```python
from build123d import *

# Parameters (mm, degrees)
F0_R     = 22.225
F1_DEPTH = 12.7
F0_R_2   = 9.525
F0_R_3   = 14.2875
F2_DEPTH = 22.225


with BuildPart() as f1:
    # F0 (on Right) → F1 (new body, symmetric)
    with BuildSketch(Plane.YZ):
        with BuildLine():
            ThreePointArc((0.7709428469, 53.3727500739), (1.3823409605, 50.5277313214), (1.5875, 47.625))
            ThreePointArc((1.5875, 47.625), (-21.5859879765, 27.1439069815), (-39.0642428209, 52.6585365854))
            ThreePointArc((-39.0642428209, 52.6585365854), (-54.8414617427, 28.4450035745), (-82.1718427428, 19.05))
            Line((-82.1718427428, 19.05), (-63.2968, 19.05))
            ThreePointArc((-63.2968, 19.05), (-44.2468, 0), (-63.2968, -19.05))
            Line((-63.2968, -19.05), (-88.6968, -19.05))
            ThreePointArc((-88.6968, -19.05), (-90.408513446, -18.9729422357), (-92.1063790378, -18.7423923442))
            Line((-92.1063790378, -18.7423923442), (-6.2508949026, -34.3610526311))
            ThreePointArc((-6.2508949026, -34.3610526311), (12.8175803312, -32.4879248253), (28.0282905638, -20.8367596586))
            ThreePointArc((28.0282905638, -20.8367596586), (37.6405240223, -14.7442138944), (48.8602257395, -16.650109833))
            ThreePointArc((48.8602257395, -16.650109833), (68.3067503871, -16.8143453506), (78.0777321497, 0))
            ThreePointArc((78.0777321497, 0), (73.3690687488, 26.7041571404), (59.8110128446, 50.1873988183))
            ThreePointArc((59.8110128446, 50.1873988183), (44.0883532808, 57.07968597), (29.0718597616, 48.7603970384))
            ThreePointArc((29.0718597616, 48.7603970384), (13.4642776808, 42.1258150573), (0.7709428469, 53.3727500739))
        make_face()
        Circle(F0_R, mode=Mode.SUBTRACT)
        with BuildLine():
            ThreePointArc((69.85, 0), (58.7248, -11.1252), (47.5996, 0))
            ThreePointArc((47.5996, 0), (44.7289928724, 16.2800220142), (36.4634090747, 30.596433106))
            ThreePointArc((36.4634090747, 30.596433106), (37.834665998, 46.2699714599), (53.5082043519, 44.8987145366))
            ThreePointArc((53.5082043519, 44.8987145366), (65.6375295619, 23.8901070113), (69.85, 0))
        make_face(mode=Mode.SUBTRACT)
    extrude(amount=F1_DEPTH, both=True)

    # F0 (on Right) → F2 (join, symmetric)
    with BuildSketch(Plane.YZ):
        with BuildLine():
            Line((-63.2968, 19.05), (-82.1718427428, 19.05))
            Line((-82.1718427428, 19.05), (-88.6968, 19.05))
            ThreePointArc((-88.6968, 19.05), (-107.6697422357, 1.711713446), (-92.1063790378, -18.7423923442))
            ThreePointArc((-92.1063790378, -18.7423923442), (-90.408513446, -18.9729422357), (-88.6968, -19.05))
            Line((-88.6968, -19.05), (-63.2968, -19.05))
            ThreePointArc((-63.2968, -19.05), (-44.2468, 0), (-63.2968, 19.05))
        make_face()
        with BuildLine():
            ThreePointArc((-88.6968, -11.0998), (-99.7966, 0), (-88.6968, 11.0998))
            Line((-88.6968, 11.0998), (-63.2968, 11.0998))
            ThreePointArc((-63.2968, 11.0998), (-52.197, 0), (-63.2968, -11.0998))
            Line((-63.2968, -11.0998), (-88.6968, -11.0998))
        make_face(mode=Mode.SUBTRACT)
        with BuildLine():
            ThreePointArc((-39.0642428209, 52.6585365854), (-21.5859879765, 27.1439069815), (1.5875, 47.625))
            ThreePointArc((1.5875, 47.625), (1.3823409605, 50.5277313214), (0.7709428469, 53.3727500739))
            ThreePointArc((0.7709428469, 53.3727500739), (-19.419954655, 68.2591837688), (-39.0642428209, 52.6585365854))
        make_face()
        with Locations((-19.05, 47.625)):
            Circle(F0_R_2, mode=Mode.SUBTRACT)
        Circle(F0_R)
        Circle(F0_R_3, mode=Mode.SUBTRACT)
    extrude(amount=F2_DEPTH, both=True)


solid = f1.part
```
The listing builds one solid part. Answer for the finished solid, in the listing's coordinates (mm). A direction names the side the tool comes from. Give positions to 0.01 mm unless a question says otherwise; leave off trailing zeros. Loops run counter-clockwise (first coordinate to the right, second up) from the corner with the lowest first, then second, coordinate; pieces in that order, holes last. Notation, with made-up numbers: (-38, 15) - (-10, 15) arc R15 ccw to (-10, 33) - close; hole circle Ø9 at (37.5, -8.75). An arc over 180 degrees is marked (long way). Return JSON: item names as keys, results as strings. Group by question number.
1. Given pin 1 Ø7.5 at (x, y) = (-9.5, -70.5) entering from +Z; pin 2 Ø6 at (y, z) = (59.5, 40.5) entering from +X; pin 3 Ø10 at (x, z) = (15, 44.5) entering from -Y; pin 4 Ø25 at (y, z) = (-19.05, 47.625) entering from +X (3 decimals), each flat-ended and moving along its own axis, determine where each tip first touches the part or whether it passes through.
2. Straight lines are drawn through the part: line 1 (Z direction, x = 13, y = 0) (1 decimal); line 2 (X direction, y = 30, z = -3); line 3 (Y direction, x = -16.5, z = -4.5). For each, find the intervals that lie inside material, in ascending order. Write a range as [from, to].
3. Determine the mould class of faces 5 (the flat face through (-22.225, -10, 43)), 6 (the cylindrical face through (-0.311, -107.742, 0.419)), 7 (the cylindrical face through (-0.311, -99.794, -0.244)), 8 (the cylindrical face through (-0.311, -14.274, 0.628)) for opening direction Y: pulls with the +Y half, pulls with the -Y half, needs draft (parallel to the pull), parting line crosses it, or undercut.
4. Find section B-B (x = 15.5). State how many separate pieces and enclosed holes the cut face has, then the cut area to 3 significant figures.
5. Find section A-A (y = 57). Write down the section's boundary in (x, z).
6. Which of the six approach directions +Z, -Z, +X, -X, +Y, -Y give full straight-line access (tool end or side, diameter ignored) to faces 1 (the cylindrical face through (-17.53, -44.25, -0.42)), 2 (the cylindrical face through (-0.311, -21.737, 68.087)), 3 (the cylindrical face through (-0.178, 58.969, -11.123)), 4 (the flat face through (17, -76, -19.05))?
7. Find section C-C (z = 6.5). Write down the section's boundary in (x, y) (3 decimals).
Verdict:
{
 "1": {"pin 1": "stops at z = 21.81", "pin 2": "stops at x = 12.7", "pin 3": "stops at y = -44.4", "pin 4": "stops at x = 22.225"},
 "2": {"line 1": "z = [-22.2, -14.3], [14.3, 22.2], [39.7, 55.6]", "line 2": "x = [-12.7, 12.7]", "line 3": "y = [-107.21, -98.84], [-53.15, -44.79], [-21.76, -13.56], [13.56, 21.76]"},
 "3": {"face 5": "needs draft", "face 6": "pulls with the -Y half", "face 7": "undercut", "face 8": "undercut"},
 "4": {"separate pieces": "3", "enclosed holes": "3", "area": "3,120 mm^2"},
 "5": {"outline": "(-12.7, -19.28) - (12.7, -19.28) - (12.7, -10.99) - (-12.7, -10.99) - close; (-12.7, 40.37) - (12.7, 40.37) - (12.7, 52.92) - (-12.7, 52.92) - close"},
 "6": {"face 1": "-X", "face 2": "none", "face 3": "+X, -X", "face 4": "-Z, +X, -Y"},
 "7": {"outline": "(-22.225, -106.604) - (22.225, -106.604) - (22.225, -97.694) - (-22.225, -97.694) - close; (-22.225, -54.299) - (22.225, -54.299) - (22.225, -45.39) - (12.7, -45.39) - (12.7, -21.253) - (22.225, -21.253) - (22.225, -12.723) - (-22.225, -12.723) - (-22.225, -21.253) - (-12.7, -21.253) - (-12.7, -45.39) - (-22.225, -45.39) - close; (-22.225, 12.723) - (22.225, 12.723) - (22.225, 21.253) - (12.7, 21.253) - (12.7, 47.154) - (-12.7, 47.154) - (-12.7, 21.253) - (-22.225, 21.253) - close; (-12.7, 69.547) - (12.7, 69.547) - (12.7, 77.807) - (-12.7, 77.807) - close"}
}
